Geometry check sheet. Reference: the model listing, model coordinates, mm. Face numbers are marked on the shaded views. Round coordinates to 2 decimals unless told otherwise and drop trailing zeros. Order: outer loops, then holes, each group sorted by start corner. A loop starts at its lowest first (then second) coordinate and runs counter-clockwise, first axis right, second up. Notation, with made-up numbers: (-39.75, -39.5) - (-11.75, -39.5) arc R31 ccw to (-11.75, -7.5) - close; hole circle Ø2 at (49, -38.75). An arc over 180 degrees is marked (long way). Write each question's results on one line, items separated by ' | '.
Autodesk Fusion 360 part; units mm, degrees
sketch "Sketch1" plane through (0, 0, 0) normal (0, 1, 0) x (1, 0, 0)
  circle A0 centre (0, 0) radius 2.5
  dimension "d1" = 5
extrude "Extrude1" add sketch "Sketch1" along normal blind 25
sketch "Sketch2" plane through (0, 25, 0) normal (0, 1, 0) x (-1, 0, 0)
  circle A0 centre (0, 0) radius 1.5
  dimension "d4" = 3
extrude "Extrude2" cut sketch "Sketch2" against normal blind 5
sketch "Sketch3" plane through (0, 0, 0) normal (0, -1, 0) x (1, 0, 0)
  circle A0 centre (0, 0) radius 1.5
  dimension "d7" = 3
extrude "Extrude3" cut sketch "Sketch3" against normal blind 5
thread "Thread1"
thread "Thread2"
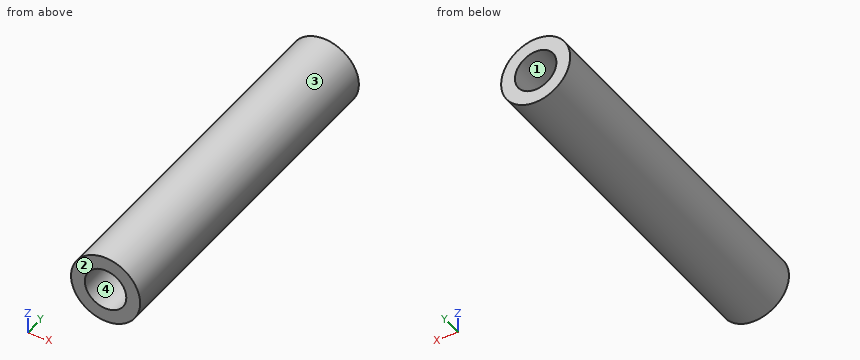
(1) Section check A-A (x = 0). Record the cut outline in (y, z).
Answers follow:
outline: (0, -2.5) - (25, -2.5) - (25, -1.5) - (20, -1.5) - (20, 1.5) - (25, 1.5) - (25, 2.5) - (0, 2.5) - (0, 1.5) - (5, 1.5) - (5, -1.5) - (0, -1.5) - close
(2) Section check C-C (y = 23.25). Record the cut outline in (x, z).
Answers follow:
outline: circle Ø5 at (0, 0); hole circle Ø3 at (0, 0)
(3) Section check D-D (y = 16). Record the cut outline in (x, z).
Answers follow:
outline: circle Ø5 at (0, 0)
(4) Section check B-B (z = 0). Record the cut outline in (x, y).
Answers follow:
outline: (-2.5, 0) - (-1.5, 0) - (-1.5, 5) - (1.5, 5) - (1.5, 0) - (2.5, 0) - (2.5, 25) - (1.5, 25) - (1.5, 20) - (-1.5, 20) - (-1.5, 25) - (-2.5, 25) - close
(5) Draft check along Z on the marked faces 1, 2, 3 and 4. Enter one of: released by +Z, released by -Z, zero draft, split by the parting line, or undercut.
Answers follow:
face 1: undercut | face 2: zero draft | face 3: split by the parting line | face 4: undercut
(6) Material ranges on line 1 (Z direction, x = 0, y = 2.05); line 2 (Y direction, x = -0.75, z = 1.05); line 3 (X direction, y = 4.5, z = 1.2), recorded low to high.
Answers follow:
line 1: -2.5 to -1.5, 1.5 to 2.5 | line 2: 5 to 20 | line 3: -2.19 to -0.9, 0.9 to 2.19
(7) Depth check by flat-ended pin: pin 1 Ø2.5 at (x, z) = (0, 0) entering from +Y; pin 2 Ø2 at (y, z) = (10, -2) entering from -X; pin 3 Ø1 at (y, z) = (4, -2) entering from -X. Enter the tip coordinate at first touch or a pass-through.
Answers follow:
pin 1: y = 20 | pin 2: x = -2.29 | pin 3: x = -2
